from build123d import *

# Parameters (mm, degrees)
SKETCH1_W           = 77.5
SKETCH1_H           = 66.8
BOSS_EXTRUDE1_DEPTH = 37.5
SKETCH3_W           = 77.5
SKETCH3_H           = 20
BOSS_EXTRUDE2_DEPTH = 2
SKETCH4_W           = 12
SKETCH4_H           = 12
BOSS_EXTRUDE3_DEPTH = 5


with BuildPart() as part:
    # Sketch1 → Boss-Extrude1 (new body)
    with BuildSketch(Plane(origin=(0, 0, 0), x_dir=(1, 0, 0), z_dir=(0, 1, 0))):
        Rectangle(SKETCH1_W, SKETCH1_H)
    extrude(amount=BOSS_EXTRUDE1_DEPTH)

    # Sketch3 → Boss-Extrude2 (add)
    with BuildSketch(Plane(origin=(0, 37.5, 0), x_dir=(1, 0, 0), z_dir=(0, 1, 0))):
        with Locations((0, -23.4)):
            Rectangle(SKETCH3_W, SKETCH3_H)
    extrude(amount=BOSS_EXTRUDE2_DEPTH)

    # Sketch4 → Boss-Extrude3 (add)
    with BuildSketch(Plane.ZY.offset(38.75)):
        with Locations((-27.4, 6)):
            Rectangle(SKETCH4_W, SKETCH4_H)
    extrude(amount=BOSS_EXTRUDE3_DEPTH)


solid = part.part
Build history of the part. All positions in model axes, mm. A direction names the side the tool comes from. Round coordinates to 2 decimals unless told otherwise and drop trailing zeros. Write each loop counter-clockwise with the first axis right and the second up, starting at its lowest first coordinate (ties: lowest second). Pieces come first, ordered by that corner, then holes. Notation, with made-up numbers: (40, 34) -> (47, 34) arc R33 ccw to (47, 73) -> close; hole circle Ø9 at (-26.75, 17.5). An arc over 180 degrees is marked (long way). Write item = value, one per line.
(1) Probe L1, parallel to X at y = 27, z = 29.5; L2, parallel to Y at x = 12, z = 7. List the from-to ranges inside material, lowest first.
Answer:
L1 = -38.75 to 38.75
L2 = 0 to 37.5
(2) Band-saw the part on B-B (z = -7.5). Give the cut face in (x, y), then the cut area to 3 significant figures.
Answer:
outline = (-38.75, 0) -> (38.75, 0) -> (38.75, 37.5) -> (-38.75, 37.5) -> close
area = 2,910 mm2
(3) Tool access for faces 1 (the face through (-41, 12, -27)), 2 (the face through (-41, 6, -21.4)), 3 (the face through (-1, 37.5, -10)): list every direction of +Z, -Z, +X, -X, +Y, -Y with a clear straight run to the whole face (end or side of a thin tool).
Answer:
face_1 = +Z, -Z, -X, +Y
face_2 = +Z, -X, +Y, -Y
face_3 = -Z, +X, -X, +Y
(4) Band-saw the part on C-C (y = 18). Give the cut face in (x, z).
Answer:
outline = (-38.75, -33.4) -> (38.75, -33.4) -> (38.75, 33.4) -> (-38.75, 33.4) -> close
(5) Band-saw the part on A-A (x = -6.5). Give the cut face in (y, z), then the cut area to 4 significant figures.
Answer:
outline = (0, -33.4) -> (37.5, -33.4) -> (37.5, 13.4) -> (39.5, 13.4) -> (39.5, 33.4) -> (0, 33.4) -> close
area = 2,545 mm2
(6) Flat gauge pins, fed straight in: pin 1 (4 mm diameter, centred on y = 33, z = -21, fed in from -X); pin 2 (2 mm diameter, centred on x = -1, y = 39, fed in from -Z); pin 3 (1.5 mm diameter, centred on x = -41, y = 7, fed in from +Z). Where does each tip first touch, or does it go through?
Answer:
pin_1 = -38.75
pin_2 = 13.4
pin_3 = -21.4
